Source: three-view drawing plus pictorial views. Frame: mm from the lowest corner of the part. A direction names the side the tool comes from. Give positions to 0.01 mm unless a question says otherwise; leave off trailing zeros. Loops run counter-clockwise (first coordinate to the right, second up) from the corner with the lowest first, then second, coordinate; pieces in that order, holes last.
1. Section A-A, the plane x = 50.5. Output: boundary loops of the cut face in (y, z) (1 decimal), then the cut area to 3 significant figures.
2. Section D-D, the plane z = 15. Output: boundary loops of the cut face in (x, y) (1 decimal).
3. Section C-C, the plane z = 24. Output: boundary loops of the cut face in (x, y) (1 decimal).
4. Draft query along X for the marked faces 1, 2 and 3. Return one class per face: +X half, -X half, draft (parallel to the pull), parting line (faces both ways), or undercut.
5. Section B-B, the plane y = 42.5. Output: boundary loops of the cut face in (x, z) (1 decimal).
6. Material intervals for line 1 along X through (y, z) = (38, 16.5) (1 decimal); line 2 along Y through (x, z) = (56, 11.5) (1 decimal), sorted ascending.
7. Access query for the marked faces 4 and 5. Directions: +Z, -Z, +X, -X, +Y, -Y. A direction counts if a zero-diameter tool reaches every point of the face in a straight line with its end or side. Return the directions, or none.
8. First-contact query: P1, Ø2.5, axis at x = 44.5, y = 48.5, coming from the +Z side. Flat tip, straight axial feed; report the tip coordinate or a pass-through.
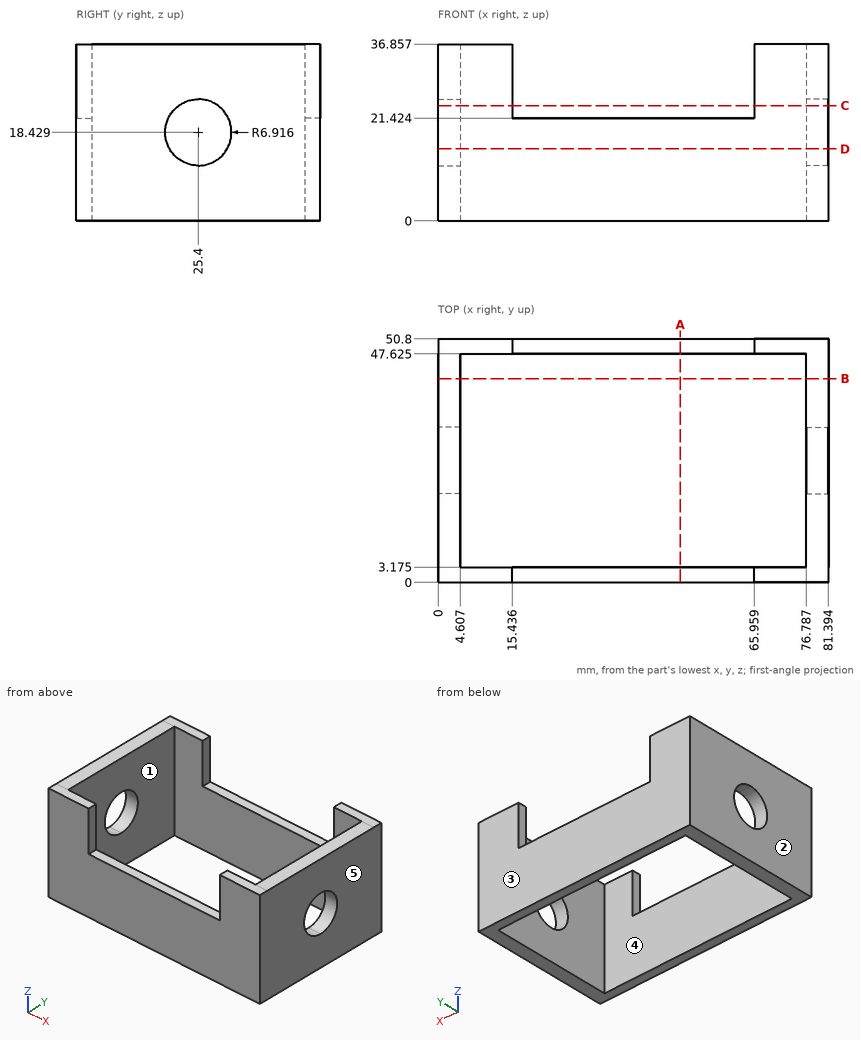
Answers below:
1. outline: (0, 0) - (3.2, 0) - (3.2, 21.4) - (0, 21.4) - close; (47.6, 0) - (50.8, 0) - (50.8, 21.4) - (47.6, 21.4) - close
1. area: 136 mm2
2. outline: (0, 0) - (81.4, 0) - (81.4, 19.4) - (76.8, 19.4) - (76.8, 3.2) - (4.6, 3.2) - (4.6, 19.4) - (0, 19.4) - close; (0, 31.4) - (4.6, 31.4) - (4.6, 47.6) - (76.8, 47.6) - (76.8, 31.4) - (81.4, 31.4) - (81.4, 50.8) - (0, 50.8) - close
3. outline: (0, 0) - (15.4, 0) - (15.4, 3.2) - (4.6, 3.2) - (4.6, 21.3) - (0, 21.3) - close; (0, 29.5) - (4.6, 29.5) - (4.6, 47.6) - (15.4, 47.6) - (15.4, 50.8) - (0, 50.8) - close; (66, 0) - (81.4, 0) - (81.4, 21.3) - (76.8, 21.3) - (76.8, 3.2) - (66, 3.2) - close; (66, 47.6) - (76.8, 47.6) - (76.8, 29.5) - (81.4, 29.5) - (81.4, 50.8) - (66, 50.8) - close
4. face 1: undercut
4. face 2: -X half
4. face 3: draft
5. outline: (0, 0) - (4.6, 0) - (4.6, 36.9) - (0, 36.9) - close; (76.8, 0) - (81.4, 0) - (81.4, 36.9) - (76.8, 36.9) - close
6. line 1: x = 0 to 4.6, 76.8 to 81.4
6. line 2: y = 0 to 3.2, 47.6 to 50.8
7. face 4: +Z, -Z
7. face 5: +Z, -Z, +X, +Y, -Y
8. P1: stops at z = 21.42
